Model file for the job. Use its own axes, mm. A direction names the side the tool comes from. Coordinates: 2 decimals unless noted, no trailing zeros. Write each loop counter-clockwise with the first axis right and the second up, starting at its lowest first coordinate (ties: lowest second). Pieces come first, ordered by that corner, then holes. Notation, with made-up numbers: (76, -23.5) - (119, -23.5) arc R19 ccw to (119, -5.5) - close; hole circle Ø4 at (21.25, 49.25). An arc over 180 degrees is marked (long way). Put each result on its own line as item: value. Start each with the question number.
1. Drop a flat-ended pin along its axis: P1, Ø0.5, axis at y = -1.5, z = 0, coming from the -X side. Give the stop position or say it passes through.
2. Which spindle directions (+Z, -Z, +X, -X, +Y, -Y) get a long thin tool onto all of the face, cutting with end or side? Do faces 5 (the face through (1, 0, -1.5)), 6 (the face through (2.176, 3.105, 1.615)). Say none if no direction does.
3. Saw through at B-B, the plane x = 1.5. Write the cut outline in (y, z).
4. Drill centre lines: L1, parallel to Y at x = 11.25, z = -1; L2, parallel to X at y = 1.5, z = 2.5; L3, parallel to Z at x = 1, y = -0.75. Where is each one in solid material? Low to high. Write a range as from..to.
5. Pull direction Y, two halves, no side cores. Call faces 1 (the face through (10, 2, 0)), 2 (the face through (4, 2, 2)), 3 (the face through (0.654, 1.293, 0.761)), 4 (the face through (1, 0, 1.5)): released by +Y, released by -Y, zero draft, split by the parting line, or undercut.
6. Saw through at A-A, the plane x = 13.25. Write the cut outline in (y, z).
```python
from build123d import *

# Parameters (mm, degrees)
FILLET1_R     = 0.1
HEX_2_DEPTH   = 1.3
CHAMFER1_SIZE = 0.3


with BuildPart() as part:
    # BodySke → Base-Revolve (revolve)
    with BuildSketch(Plane.XY, mode=Mode.PRIVATE) as base_revolve_sk:
        Polygon((0, 0), (0, 3.5), (4, 3.5), (4, 2), (15.7195, 2), (16, 1.7195), (16, 0), align=None)
    revolve(base_revolve_sk.sketch.rotate(Axis((-31.75, 0, 0), (1, 0, 0)), 90), axis=Axis((-31.75, 0, 0), (1, 0, 0)))

    # Fillet1
    fillet1_edges = [part.edges().sort_by_distance(p)[0] for p in [
        (4, 0, -2),
    ]]
    fillet(fillet1_edges, radius=FILLET1_R)

    # Sketch2 → Hex-PreBroach (revolve, cut)
    with BuildSketch(Plane.XY, mode=Mode.PRIVATE) as hex_prebroach_sk:
        Polygon((0, 1.5), (1.3, 1.5), (2.166025404, 0), (0, 0), align=None)
    revolve(hex_prebroach_sk.sketch.rotate(Axis((0, 0, 0), (1, 0, 0)), 90), axis=Axis((0, 0, 0), (1, 0, 0)), mode=Mode.SUBTRACT)

    # Sketch3 → Hex 2 (cut)
    with BuildSketch(Plane(origin=(0, 0, 0), x_dir=(0, 0.500000000000001, 0.866025403784438), z_dir=(-1, 0, 0))):
        Polygon((0.866025404, 1.5), (-0.866025404, 1.5), (-1.732050808, 0), (-0.866025404, -1.5), (0.866025404, -1.5), (1.732050808, 0), align=None)
    extrude(amount=-HEX_2_DEPTH, mode=Mode.SUBTRACT)

    # Chamfer1
    chamfer1_edges = [part.edges().sort_by_distance(p)[0] for p in [
        (0, 0, -3.5),
    ]]
    chamfer(chamfer1_edges, length=CHAMFER1_SIZE)

    # Sketch4 → Cut-Revolve1 (revolve, cut)
    with BuildSketch(Plane(origin=(0, 0, 0), x_dir=(1, 0, 0), z_dir=(0, 1, 0))):
        Polygon((0, 1.778), (1.026528779, 0), (0, 0), align=None)
    revolve(axis=Axis((1.026528779, 0, 0), (1, 0, 0)), mode=Mode.SUBTRACT)


solid = part.part
```
Final values:
1. P1: stops at x = 0.02
2. face 5: -X
2. face 6: +X, -X
3. outline: circle Ø7 at (0, 0); hole circle Ø2.31 at (0, 0)
4. L1: y = -1.73..1.73
4. L2: x = 0..4
4. L3: z = -3.42..-1.5, 1.5..3.42
5. face 1: split by the parting line
5. face 2: zero draft
5. face 3: undercut
5. face 4: undercut
6. outline: circle Ø4 at (0, 0)
